Design review of the part built by this model. Coordinates are the model's own, in mm. Coordinates: 2 decimals unless noted, no trailing zeros. Write each loop counter-clockwise with the first axis right and the second up, starting at its lowest first coordinate (ties: lowest second). Pieces come first, ordered by that corner, then holes.
Q1. Take a section at B-B (x = 74). Give the boundary of the cut face in (y, z).
Q2. Insertion check: pin 1 (1 mm diameter, centred on x = 82.5, y = 32.5, fed in from +Z); pin 2 (1.5 mm diameter, centred on x = 78.5, y = 60.5, fed in from +Z) (1 decimal). Each pin has a flat end and moves straight along its axis. Give the tip position at first contact, or say it passes through.
Q3. Take a section at A-A (y = 8.5). Give the boundary of the cut face in (x, z), and give its area (3 significant figures).
Q4. Take a section at C-C (z = 0.1). State how many separate pieces and enclosed holes the cut face has, and give its area (3 significant figures).
Q5. For probe 1 along X at (y, z) = (0, 0.15) (3 decimals); probe 2 along Y at (x, z) = (66, 0.2); probe 3 along X at (y, z) = (9, 0.2), list the stretches that pass through material, from the lowest coordinate up.
Q6. Take a section at D-D (x = 38). Give the boundary of the cut face in (y, z), and give its area (3 significant figures).
```python
from build123d import *

# Parameters (mm, degrees)
BOSS_EXTRUDE1_DEPTH = 0.254
SKETCH2_R           = 4.699
CUT_EXTRUDE1_DEPTH  = 1.254
SKETCH3_W           = 2.54
SKETCH3_H           = 0.635
CUT_EXTRUDE2_DEPTH  = 1.254
CUT_EXTRUDE3_DEPTH  = 1.254


with BuildPart() as part:
    # Sketch1 → Boss-Extrude1 (new body)
    with BuildSketch(Plane.XY):
        with BuildLine():
            Line((27.218819563, 62.393373411), (22.357699804, 50.65759216))
            ThreePointArc((22.357699804, 50.65759216), (28.61353693, 47.405947816), (34.405475059, 43.38573118))
            Line((34.405475059, 43.38573118), (8.696654013, 17.676910134))
            Line((8.696654013, 17.676910134), (7.228954972, 14.133571205))
            ThreePointArc((7.228954972, 14.133571205), (14.666587579, 6.075099489), (15.105587123, -4.88230096))
            Line((15.105587123, -4.88230096), (18.648926052, -6.35))
            Line((18.648926052, -6.35), (101.401368334, -6.35))
            ThreePointArc((101.401368334, -6.35), (93.866160503, 38.880636728), (67.21146711, 76.191723231))
            Line((67.21146711, 76.191723231), (43.43415954, 52.414415661))
            ThreePointArc((43.43415954, 52.414415661), (35.677104191, 57.973626939), (27.218819563, 62.393373411))
        make_face()
        with BuildLine():
            Line((88.672924278, 6.35), (27.86051193, 6.35))
            ThreePointArc((27.86051193, 6.35), (26.399857642, 10.93517908), (24.190484974, 15.210228852))
            Line((24.190484974, 15.210228852), (67.191354125, 58.211098004))
            ThreePointArc((67.191354125, 58.211098004), (82.13289044, 34.020557137), (88.672924278, 6.35))
        make_face(mode=Mode.SUBTRACT)
    extrude(amount=BOSS_EXTRUDE1_DEPTH)

    # Sketch2 → Cut-Extrude1 (cut, through all)
    with BuildSketch(Plane.XY.offset(0.254)):
        with Locations((22.225, 0)):
            Circle(SKETCH2_R)
        with Locations((36.195, 0)):
            Circle(SKETCH2_R)
        with Locations((61.722, 0)):
            Circle(SKETCH2_R)
        with Locations((75.692, 0)):
            Circle(SKETCH2_R)
        with Locations((95.25, 0)):
            Circle(SKETCH2_R)
        with Locations((15.715448212, 15.715448212)):
            Circle(SKETCH2_R)
        with Locations((25.593729945, 25.593729945)):
            Circle(SKETCH2_R)
        with Locations((43.644044748, 43.644044748)):
            Circle(SKETCH2_R)
        with Locations((53.522326482, 53.522326482)):
            Circle(SKETCH2_R)
        with Locations((92.004434954, 24.652514046)):
            Circle(SKETCH2_R)
        with Locations((82.48891971, 47.625)):
            Circle(SKETCH2_R)
        with Locations((67.351920908, 67.351920908)):
            Circle(SKETCH2_R)
        with Locations((30.861, 53.452819972)):
            Circle(SKETCH2_R)
    extrude(amount=-CUT_EXTRUDE1_DEPTH, mode=Mode.SUBTRACT)

    # Sketch3 → Cut-Extrude2 (cut, through all)
    with BuildSketch(Plane.XY.offset(0.254)):
        Polygon((15.266435406, 24.246691527), (17.06248663, 26.042742751), (17.511499436, 25.593729945), (15.715448212, 23.797678721), align=None)
        Polygon((43.43415954, 52.414415661), (44.991083167, 53.971339288), (45.440095973, 53.522326482), (43.883172346, 51.965402855), align=None)
        with Locations((29.21, -6.0325)):
            Rectangle(SKETCH3_W, SKETCH3_H)
        with Locations((68.707, -6.0325)):
            Rectangle(SKETCH3_W, SKETCH3_H)
        Polygon((29.230733674, 38.210989795), (31.026784898, 40.007041019), (31.475797704, 39.558028213), (29.67974648, 37.761976989), align=None)
        Polygon((56.845021246, 65.825277367), (55.048970022, 64.029226143), (55.497982828, 63.580213337), (57.294034052, 65.376264561), align=None)
        with Locations((48.9585, -6.0325)):
            Rectangle(SKETCH3_W, SKETCH3_H)
        with Locations((85.471, -6.0325)):
            Rectangle(SKETCH3_W, SKETCH3_H)
        Polygon((99.935462164, 14.437711971), (100.266998693, 11.919442024), (101.526133667, 12.085210288), (101.194597138, 14.603480236), align=None)
        Polygon((93.765504959, 37.464305742), (94.938831965, 37.950313702), (93.966816047, 40.296967714), (92.793489041, 39.810959755), align=None)
        Polygon((79.327792988, 62.471156422), (80.874047017, 60.456038938), (81.88160576, 61.229165953), (80.33535173, 63.244283437), align=None)
        Polygon((13.593916116, 7.005422516), (14.565932035, 4.658768503), (15.739259041, 5.144776462), (14.767243123, 7.491430475), align=None)
    extrude(amount=-CUT_EXTRUDE2_DEPTH, mode=Mode.SUBTRACT)

    # Sketch7 → Cut-Extrude3 (cut, through all)
    with BuildSketch(Plane.XY.offset(0.254)):
        with BuildLine():
            Line((12.392753447, 19.038142977), (22.27103518, 28.91642471))
            ThreePointArc((22.27103518, 28.91642471), (28.91642471, 28.91642471), (28.91642471, 22.27103518))
            Line((28.91642471, 22.27103518), (19.038142977, 12.392753447))
            ThreePointArc((19.038142977, 12.392753447), (12.392753447, 12.392753447), (12.392753447, 19.038142977))
        make_face()
        with BuildLine():
            Line((22.225, 4.699), (36.195, 4.699))
            ThreePointArc((36.195, 4.699), (40.894, 0), (36.195, -4.699))
            Line((36.195, -4.699), (22.225, -4.699))
            ThreePointArc((22.225, -4.699), (17.526, 0), (22.225, 4.699))
        make_face()
        with BuildLine():
            Line((61.722, 4.699), (75.692, 4.699))
            ThreePointArc((75.692, 4.699), (80.391, 0), (75.692, -4.699))
            Line((75.692, -4.699), (61.722, -4.699))
            ThreePointArc((61.722, -4.699), (57.023, 0), (61.722, 4.699))
        make_face()
        with BuildLine():
            ThreePointArc((46.966739513, 46.966739513), (40.434542876, 52.695322215), (33.2105, 57.522273345))
            ThreePointArc((33.2105, 57.522273345), (26.791546628, 55.802319972), (28.5115, 49.3833666))
            ThreePointArc((28.5115, 49.3833666), (34.713402966, 45.239387523), (40.321349984, 40.321349984))
            ThreePointArc((40.321349984, 40.321349984), (46.966739513, 40.321349984), (46.966739513, 46.966739513))
        make_face()
        with BuildLine():
            ThreePointArc((99.949, 0), (99.093922449, 13.045962386), (96.543320412, 25.868704739))
            ThreePointArc((96.543320412, 25.868704739), (90.788244261, 29.191399504), (87.465549496, 23.436323353))
            ThreePointArc((87.465549496, 23.436323353), (89.776323642, 11.819277232), (90.551, 0))
            ThreePointArc((90.551, 0), (95.25, -4.699), (99.949, 0))
        make_face()
        with BuildLine():
            ThreePointArc((86.558373083, 49.9745), (79.294873009, 60.845096068), (70.674615673, 70.674615673))
            ThreePointArc((70.674615673, 70.674615673), (64.029226143, 70.674615673), (64.029226143, 64.029226143))
            ThreePointArc((64.029226143, 64.029226143), (71.838938317, 55.123956158), (78.419466338, 45.2755))
            ThreePointArc((78.419466338, 45.2755), (84.83841971, 43.555546628), (86.558373083, 49.9745))
        make_face()
    extrude(amount=-CUT_EXTRUDE3_DEPTH, mode=Mode.SUBTRACT)


solid = part.part
```
Response:
1. outline: (-6.35, 0) - (-4.7, 0) - (-4.7, 0.25) - (-6.35, 0.25) - close; (4.7, 0) - (6.35, 0) - (6.35, 0.25) - (4.7, 0.25) - close; (49.27, 0) - (52.19, 0) - (52.19, 0.25) - (49.27, 0.25) - close; (67.18, 0) - (69.62, 0) - (69.62, 0.25) - (67.18, 0.25) - close
2. pin 1: stops at z = 0.25
2. pin 2: passes through
3. outline: (13.41, 0) - (27.28, 0) - (27.28, 0.25) - (13.41, 0.25) - close; (88.49, 0) - (90.15, 0) - (90.15, 0.25) - (88.49, 0.25) - close; (99.59, 0) - (101.24, 0) - (101.24, 0.25) - (99.59, 0.25) - close
3. area: 4.37 mm2
4. separate pieces: 1
4. enclosed holes: 8
4. area: 1,720 mm2
5. probe 1: x = 15.875 to 17.526, 40.894 to 57.023, 80.391 to 90.551, 99.949 to 101.6
5. probe 2: y = -6.35 to -4.7, 4.7 to 6.35, 57.02 to 62, 71.85 to 74.98
5. probe 3: x = 13.08 to 27.12, 88.44 to 90.1, 99.54 to 101.2
6. outline: (-6.35, 0) - (-4.34, 0) - (-4.34, 0.25) - (-6.35, 0.25) - close; (4.34, 0) - (6.35, 0) - (6.35, 0.25) - (4.34, 0.25) - close; (29.02, 0) - (42.52, 0) - (42.52, 0.25) - (29.02, 0.25) - close; (54.48, 0) - (56.48, 0) - (56.48, 0.25) - (54.48, 0.25) - close
6. area: 4.96 mm2
